Part model, mm, in its own coordinate system. A direction names the side the tool comes from. Give positions to 0.01 mm unless a question says otherwise; leave off trailing zeros. Write each loop counter-clockwise with the first axis right and the second up, starting at its lowest first coordinate (ties: lowest second). Pieces come first, ordered by that corner, then holes. Notation, with made-up numbers: M -19.75,5 L -8.75,5 A28 ccw -8.75,27 Z; hole C 17,-14 d2. An arc over 180 degrees is marked long. Use CSV: the item, a comma, the result in double quotes. Start each with the question number.
Item 1: Pin check, flat tips, straight feed: pin 1 (12 mm diameter, centred on x = -172.5, y = -103, fed in from -Z); pin 2 (9 mm diameter, centred on x = 500.5, y = -131.5, fed in from +Z); pin 3 (4 mm diameter, centred on x = 9.5, y = -74, fed in from +Z). Stop position of each tip, or through.
Item 2: Cut at B-B (x = 52). List the corners of the cut face in (y, z), then the cut area to 3 significant figures.
Item 3: Which spindle directions (+Z, -Z, +X, -X, +Y, -Y) get a long thin tool onto all of the face, cutting with end or side? Do faces 1 (the flat face through (481.983, 233, -158)), 2 (the flat face through (481.983, -150, -323)), 3 (the flat face through (-478.017, 233, -424)), 4 (the flat face through (-493, 218.136, -424)), 5 (the flat face through (-493, -321.864, -158)). Say none if no direction does.
Item 4: Cut at C-C (y = 197.5). List the corners of the cut face in (x, z).
Item 5: Cut at D-D (y = -181.5). List the corners of the cut face in (x, z).
Item 6: Mould opens along Z. For faces 6 (the flat face through (-493, 233, -500)), 7 (the flat face through (481.983, 233, -424)), 8 (the flat face through (-493, -56, -320)) say: released by +Z, released by -Z, zero draft, split by the parting line, or undercut.
Item 7: Cut at A-A (z = -127.5). List the corners of the cut face in (x, y).
Item 8: Drill centre lines: line 1 (X direction, y = 146, z = 67.5); line 2 (X direction, y = 219.5, z = -231.5); line 3 (Y direction, x = -188, z = 64.5). Where is each one in solid material? Low to high. Write a range as [from, to].
from build123d import *

# Parameters (mm, degrees)
F0_W      = 1020
F0_H      = 600
F1_DEPTH  = 30
F3_DEPTH  = 150
F5_DEPTH  = 2000
F6_W      = 30
F6_H      = 30
F7_DEPTH  = 500
F8_W      = 30
F8_H      = 30
F9_DEPTH  = 540
F10_W     = 30
F10_H     = 30
F11_DEPTH = 540
F12_W     = 30
F12_H     = 30
F13_DEPTH = 960


with BuildPart() as f1:
    # F0 (on Top) → F1 (new body)
    with BuildSketch(Plane.XY):
        with Locations((1.982912, -51.863651)):
            Rectangle(F0_W, F0_H)
    extrude(amount=F1_DEPTH)

    # F2 (on face) → F3 (join)
    with BuildSketch(Plane.XY.offset(30)):
        Polygon((-508.017088, 248.136349), (-508.017088, -351.863651), (-488.017088, -351.863651), (-488.017088, 228.136349), (491.982912, 228.136349), (491.982912, -351.863651), (511.982912, -351.863651), (511.982912, 248.136349), align=None)
    extrude(amount=F3_DEPTH)

    # F4 (on face) → F5 (cut)
    with BuildSketch(Plane(origin=(-508.017088, 0, 0), x_dir=(0, -1, 0), z_dir=(-1, 0, 0))):
        Polygon((351.863651, 180), (-218.136349, 180), (351.863651, 50), align=None)
    extrude(amount=-F5_DEPTH, mode=Mode.SUBTRACT)

    # F6 (on face) → F7 (join)
    with BuildSketch(Plane(origin=(0, 0, 0), x_dir=(1, 0, 0), z_dir=(0, 0, -1))):
        with Locations((-493.017088, 336.863651)):
            Rectangle(F6_W, F6_H)
        with Locations((-493.017088, -233.136349)):
            Rectangle(F6_W, F6_H)
        with Locations((496.982912, 336.863651)):
            Rectangle(F6_W, F6_H)
        with Locations((496.982912, -233.136349)):
            Rectangle(F6_W, F6_H)
    extrude(amount=F7_DEPTH)

    # F8 (on face) → F9 (join, through all)
    with BuildSketch(Plane(origin=(0, -321.863651, 0), x_dir=(-1, 0, 0), z_dir=(0, 1, 0))):
        with Locations((493.017088, -335)):
            Rectangle(F8_W, F8_H)
    extrude(amount=F9_DEPTH)

    # F10 (on face) → F11 (join, through all)
    with BuildSketch(Plane.XZ.offset(-218.136349)):
        with Locations((496.982912, -335)):
            Rectangle(F10_W, F10_H)
    extrude(amount=F11_DEPTH)

    # F12 (on face) → F13 (join, through all)
    with BuildSketch(Plane(origin=(481.982912, 0, 0), x_dir=(0, -1, 0), z_dir=(-1, 0, 0))):
        with Locations((-233.136349, -335)):
            Rectangle(F12_W, F12_H)
    extrude(amount=F13_DEPTH)


solid = f1.part
Worked answers:
1,pin 1,"stops at z = 0"
1,pin 2,"stops at z = 101.28"
1,pin 3,"stops at z = 30"
2,outline,"M -351.86,0 L 248.14,0 L 248.14,180 L 228.14,180 L 228.14,30 L -351.86,30 Z; M 218.14,-350 L 248.14,-350 L 248.14,-320 L 218.14,-320 Z"
2,area,"21,900 mm^2"
3,face 1,"+Y, -Y"
3,face 2,"-Z, -Y"
3,face 3,"-Z, +Y, -Y"
3,face 4,"-Z, +X, -X"
3,face 5,"+X, -X"
4,outline,"M -508.02,-350 L -478.02,-350 L -478.02,-320 L -508.02,-320 Z; M -508.02,0 L 511.98,0 L 511.98,175.29 L 491.98,175.29 L 491.98,30 L -488.02,30 L -488.02,175.29 L -508.02,175.29 Z; M 481.98,-350 L 511.98,-350 L 511.98,-320 L 481.98,-320 Z"
5,outline,"M -508.02,-350 L -478.02,-350 L -478.02,-320 L -508.02,-320 Z; M -508.02,0 L 511.98,0 L 511.98,88.85 L 491.98,88.85 L 491.98,30 L -488.02,30 L -488.02,88.85 L -508.02,88.85 Z; M 481.98,-350 L 511.98,-350 L 511.98,-320 L 481.98,-320 Z"
6,face 6,"released by -Z"
6,face 7,"zero draft"
6,face 8,"undercut"
7,outline,"M -508.02,-351.86 L -478.02,-351.86 L -478.02,-321.86 L -508.02,-321.86 Z; M -508.02,218.14 L -478.02,218.14 L -478.02,248.14 L -508.02,248.14 Z; M 481.98,-351.86 L 511.98,-351.86 L 511.98,-321.86 L 481.98,-321.86 Z; M 481.98,218.14 L 511.98,218.14 L 511.98,248.14 L 481.98,248.14 Z"
8,line 1,"x = [-508.02, -488.02], [491.98, 511.98]"
8,line 2,"x = [-508.02, -478.02], [481.98, 511.98]"
8,line 3,"y = [228.14, 248.14]"
